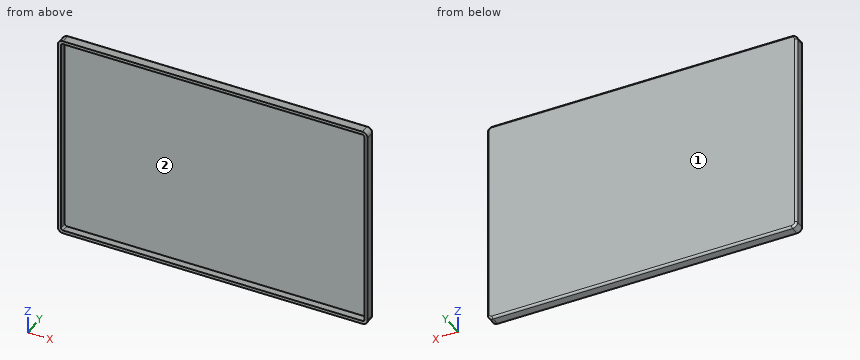
```python
from build123d import *

# Parameters (mm, degrees)
BOSS_EXTRUDE1_DEPTH = 10
SHELL1_T            = -3
FILLET1_R           = 2


with BuildPart() as part:
    # Sketch1 → Boss-Extrude1 (new body)
    with BuildSketch(Plane(origin=(0, 0, 0), x_dir=(1, 0, 0), z_dir=(0, 1, 0))):
        with BuildLine():
            Line((-145, 100), (145, 100))
            ThreePointArc((145, 100), (148.535533906, 98.535533906), (150, 95))
            Line((150, 95), (150, -95))
            ThreePointArc((150, -95), (148.535533906, -98.535533906), (145, -100))
            Line((145, -100), (-145, -100))
            ThreePointArc((-145, -100), (-148.535533906, -98.535533906), (-150, -95))
            Line((-150, -95), (-150, 95))
            ThreePointArc((-150, 95), (-148.535533906, 98.535533906), (-145, 100))
        make_face()
    extrude(amount=BOSS_EXTRUDE1_DEPTH)

    # Shell1
    shell1_openings = [part.faces().sort_by_distance(p)[0] for p in [
        (0, 0, 0),
    ]]
    offset(amount=SHELL1_T, openings=shell1_openings, kind=Kind.INTERSECTION)

    # Fillet1
    fillet1_edges = [part.edges().sort_by_distance(p)[0] for p in [
        (-148.535533906, 10, -98.535533906),
        (-150, 10, 0),
        (-148.535533906, 10, 98.535533906),
        (0, 10, 100),
        (148.535533906, 10, 98.535533906),
        (150, 10, 0),
        (148.535533906, 10, -98.535533906),
        (0, 10, -100),
    ]]
    fillet(fillet1_edges, radius=FILLET1_R)


solid = part.part
```
Geometry: final body of the model. Coordinates: model frame, mm. Face numbers are marked on the shaded views. Give positions to 0.01 mm unless a question says otherwise; leave off trailing zeros. Loops run counter-clockwise (first coordinate to the right, second up) from the corner with the lowest first, then second, coordinate; pieces in that order, holes last. Notation, with made-up numbers: (43.5, -34) -> (68.5, -34) arc R25 cw to (68.5, -9) -> close; hole circle Ø10 at (34.5, 25). An arc over 180 degrees is marked (long way). Return JSON: item names as keys, results as strings.
Item 1: Section C-C, the plane z = 54. Output: boundary loops of the cut face in (x, y), plus the area to 3 significant figures.
Filled in:
{"outline": "(-150, 0) -> (-147, 0) -> (-147, 7) -> (147, 7) -> (147, 0) -> (150, 0) -> (150, 8) arc R2 ccw to (148, 10) -> (-148, 10) arc R2 ccw to (-150, 8) -> close", "area": "940 mm^2"}
Item 2: Section B-B, the plane x = 70.5. Output: boundary loops of the cut face in (y, z), plus the area to 3 significant figures.
Filled in:
{"outline": "(0, -100) -> (8, -100) arc R2 ccw to (10, -98) -> (10, 98) arc R2 ccw to (8, 100) -> (0, 100) -> (0, 97) -> (7, 97) -> (7, -97) -> (0, -97) -> close", "area": "640 mm^2"}
Item 3: Section A-A, the plane y = 4.25. Output: boundary loops of the cut face in (x, z), plus the area to 3 significant figures.
Filled in:
{"outline": "(-150, -95) arc R5 ccw to (-145, -100) -> (145, -100) arc R5 ccw to (150, -95) -> (150, 95) arc R5 ccw to (145, 100) -> (-145, 100) arc R5 ccw to (-150, 95) -> close; hole (-147, -95) arc R2 ccw to (-145, -97) -> (145, -97) arc R2 ccw to (147, -95) -> (147, 95) arc R2 ccw to (145, 97) -> (-145, 97) arc R2 ccw to (-147, 95) -> close", "area": "2,950 mm^2"}
Item 4: Mould query, pull axis Z, two halves, no side actions, for the marked faces 1 and 2. Classes: released by +Z, released by -Z, zero draft, split by the parting line, or undercut.
Filled in:
{"face 1": "zero draft", "face 2": "undercut"}
Item 5: Line query: line 1 (Z direction, x = -3, y = 5.5); line 2 (X direction, y = 2, z = -82); line 3 (Z direction, x = -44, y = 8.5). Output: solid intervals per line, ascending.
Filled in:
{"line 1": "-100 to -97, 97 to 100", "line 2": "-150 to -147, 147 to 150", "line 3": "-99.94 to 99.94"}
Item 6: Pin query (flat end, axial travel): P1, Ø2, axis at x = 48, z = -28, coming from the -Y side. Return the tip coordinate at first contact, or that it passes through.
Filled in:
{"P1": "y = 7"}
